Work out the finished part from the listing and answer in its coordinate system (mm). A direction names the side the tool comes from. Coordinates: 2 decimals unless noted, no trailing zeros. Order: outer loops, then holes, each group sorted by start corner. A loop starts at its lowest first (then second) coordinate and runs counter-clockwise, first axis right, second up. Notation, with made-up numbers: (-16, 26.5) - (18, 26.5) arc R24 cw to (18, 37.5) - close; hole circle Ø10 at (17, 34). An arc over 180 degrees is marked (long way). Use CSV: the item, a comma, the result in double quotes. Start each with the question number.
from build123d import *

# Parameters (mm, degrees)
SKETCH006_R             = 1.5
SKETCH006_R_2           = 1.75
PAD002_DEPTH            = 3
FILLET_R                = 1
SKETCH_R                = 3.05
POCKET_DEPTH            = 1.8
BODY001_PLACEMENT_ANGLE = 180


with BuildPart() as part:
    # Sketch006 → Pad002 (new body)
    with BuildSketch(Plane.XY):
        with BuildLine():
            Line((5, 0), (56.76, 0))
            ThreePointArc((56.76, 0), (68.285841, 4.774159), (73.06, 16.3))
            ThreePointArc((73.06, 16.3), (72.202439, 19.100036), (69.92392, 20.939591))
            Line((48.183063, 29.673815), (69.92392, 20.939591))
            ThreePointArc((48.183063, 38.952996), (45.046983, 34.313406), (48.183063, 29.673815))
            Line((48.183063, 38.952996), (66.196084, 46.189591))
            ThreePointArc((68.060005, 46.55), (67.110782, 46.459071), (66.196084, 46.189591))
            Line((68.060005, 46.55), (93.060005, 46.55))
            Line((93.060005, 51.55), (93.060005, 46.55))
            Line((93.060005, 56.55), (93.060005, 51.55))
            Line((93.060005, 56.55), (28.06, 56.55))
            ThreePointArc((28.06, 56.55), (26.826846, 56.395547), (25.669877, 55.941732))
            Line((2.609877, 43.391732), (25.669877, 55.941732))
            ThreePointArc((2.609877, 43.391732), (0.701709, 41.554348), (0, 39))
            Line((0, 39), (0, 5))
            ThreePointArc((0, 5), (1.464466, 1.464466), (5, 0))
        make_face()
        with Locations((5, 5)):
            Circle(SKETCH006_R, mode=Mode.SUBTRACT)
        with Locations((39, 5)):
            Circle(SKETCH006_R, mode=Mode.SUBTRACT)
        with Locations((39, 39)):
            Circle(SKETCH006_R, mode=Mode.SUBTRACT)
        with Locations((5, 39)):
            Circle(SKETCH006_R, mode=Mode.SUBTRACT)
        with Locations((28.06, 51.55)):
            Circle(SKETCH006_R_2, mode=Mode.SUBTRACT)
        with Locations((68.06, 51.55)):
            Circle(SKETCH006_R_2, mode=Mode.SUBTRACT)
        with Locations((68.06, 16.3)):
            Circle(SKETCH006_R_2, mode=Mode.SUBTRACT)
        with Locations((28.06, 16.3)):
            Circle(SKETCH006_R_2, mode=Mode.SUBTRACT)
        with BuildLine():
            ThreePointArc((38.06, 53.3), (36.31, 51.55), (38.06, 49.8))
            Line((38.06, 49.8), (58.06, 49.8))
            ThreePointArc((58.06, 49.8), (59.81, 51.55), (58.06, 53.3))
            Line((38.06, 53.3), (58.06, 53.3))
        make_face(mode=Mode.SUBTRACT)
        with BuildLine():
            ThreePointArc((78.06, 53.3), (76.31, 51.55), (78.06, 49.8))
            Line((78.06, 49.8), (84.810005, 49.8))
            ThreePointArc((84.810005, 49.8), (86.560005, 51.55), (84.810005, 53.3))
            Line((78.06, 53.3), (84.810005, 53.3))
        make_face(mode=Mode.SUBTRACT)
    extrude(amount=PAD002_DEPTH)

    # Fillet
    fillet_edges = [part.edges().sort_by_distance(p)[0] for p in [
        (93.060005, 46.55, 1.5),
        (93.060005, 56.55, 1.5),
    ]]
    fillet(fillet_edges, radius=FILLET_R)

    # Sketch (on Face2 of Fillet) → Pocket (cut)
    with BuildSketch(Plane(origin=(0, 0, 0), x_dir=(1, 0, 0), z_dir=(0, 0, -1))):
        with Locations((5, -5)):
            Circle(SKETCH_R)
        with Locations((39, -5)):
            Circle(SKETCH_R)
        with Locations((39, -39)):
            Circle(SKETCH_R)
        with Locations((5, -39)):
            Circle(SKETCH_R)
    extrude(amount=-POCKET_DEPTH, mode=Mode.SUBTRACT)


with BuildPart() as part_1:
    # Body001 placement: moved
    add(part.part.moved(Location((0.94, 56.55, 3))).rotate(Axis((0.94, 56.55, 3), (1, 0, 0)), BODY001_PLACEMENT_ANGLE))


solid = part_1.part
1) For faces 4 (the face through (37.25, 4.96, 1.52)), 5 (the face through (1.661, 14.963, 1.521)), 6 (the face through (36, 28, 3)), 7 (the face through (81, 10, 2)), 8 (the face through (5.279, 14.573, 2.113)), determine the directions among +Z, -Z, +X, -X, +Y, -Y from which every point of the face is accessible in a straight line to the end or side of a thin tool.
2) The part is cut by section B-B on x = 83.5. Determine the outline of the cut face in (y, z), plus the area to 3 significant figures.
3) The part is cut by section D-D on x = 25. Determine the outline of the cut face in (y, z).
4) The part is cut by section C-C on y = 5. Determine the outline of the cut face in (x, z).
5) The part is cut by section A-A on z = 2. State how many separate pieces and enclosed holes the cut face has, plus the area to 3 significant figures.
6) For a pull along X with two mould halves and no side action, classify faces 1 (the face through (38.83, 50.54, 0.61)), 2 (the face through (31, 56.55, 2)), 3 (the face through (59.84, 31.18, 1.52)) as +X half, -X half, draft (parallel to the pull), parting line (faces both ways), or undercut.
7) Flat-ended cylindrical pins translate along their axes: P1, Ø2.5, axis at x = 5.94, y = 51.55, coming from the -Z side; P2, Ø3.5, axis at x = 5.94, y = 17.55, coming from the +Z side; P3, Ø1, axis at y = 47, z = 1, coming from the +X side. Find the tip coordinate at first contact, or state that the pin passes through.
8) Straight lines are drawn through the part: line 1 (X direction, y = 40.25, z = 2); line 2 (Y direction, x = 29, z = 1.4); line 3 (Y direction, x = 39.94, z = 2.4). For each, find the intervals that lie inside material, in ascending order. Write a range as [from, to].
Answer key:
1,face 4,"+Z, -Z"
1,face 5,"+Z, -Z, -X, -Y"
1,face 6,"+Z, +X, -X, +Y, -Y"
1,face 7,"+Z, -Z, +X"
1,face 8,"+Z"
2,outline,"(0, 0) - (3.25, 0) - (3.25, 3) - (0, 3) - close; (6.75, 0) - (10, 0) - (10, 3) - (6.75, 3) - close"
2,area,"19.5 mm^2"
3,outline,"(1.48, 0) - (56.55, 0) - (56.55, 3) - (1.48, 3) - close"
4,outline,"(18.54, 0) - (27.25, 0) - (27.25, 3) - (18.54, 3) - close; (30.75, 0) - (37.25, 0) - (37.25, 3) - (30.75, 3) - close; (60.75, 0) - (67.25, 0) - (67.25, 3) - (60.75, 3) - close; (70.75, 0) - (77.25, 0) - (77.25, 3) - (70.75, 3) - close; (87.5, 0) - (94, 0) - (94, 3) - (87.5, 3) - close"
5,separate pieces,"1"
5,enclosed holes,"10"
5,area,"3,310 mm^2"
6,face 1,"undercut"
6,face 2,"draft"
6,face 3,"+X half"
7,P1,"through"
7,P2,"z = 1.2"
7,P3,"x = 72.75"
8,line 1,"[0.94, 27.25], [30.75, 67.25], [70.75, 74]"
8,line 2,"[0, 3.25], [6.75, 38.5], [42, 56.55]"
8,line 3,"[0, 3.25], [6.75, 14.5], [20.6, 48.5], [54.6, 56.55]"
